Can you work these out from the model? Positions are in its coordinate system, mm. Face numbers are marked on the shaded views. A direction names the side the tool comes from. Give positions to 0.01 mm unless a question says otherwise; leave off trailing zeros. Loops run counter-clockwise (first coordinate to the right, second up) from the corner with the lowest first, then second, coordinate; pieces in that order, holes last. Notation, with made-up numbers: (-23, 85) -> (5, 85) arc R17 ccw to (5, 94) -> close; hole circle Ø11 at (47.5, 20.25). An arc over 180 degrees is marked (long way). Use CSV: the item, a comma, the result in double quotes.
from build123d import *

# Parameters (mm, degrees)
BOSS_EXTRUDE1_DEPTH       = 3
SKETCH2_W                 = 10
SKETCH2_H                 = 4.5
BOSS_EXTRUDE2_DEPTH       = 5
M2X0_4_TAPPED_HOLE1_D     = 1.6
M2X0_4_TAPPED_HOLE1_DEPTH = 5.2
M2X0_4_TAPPED_HOLE1_TIP   = 0.480688495
M3X0_5_TAPPED_HOLE1_D     = 2.5
M14_CLEARANCE_HOLE1_D     = 16
FILLET1_R                 = 1.749999932


with BuildPart() as part:
    # Sketch1 → Boss-Extrude1 (new body)
    with BuildSketch(Plane.XZ):
        with BuildLine():
            Line((-5, 5.422252789), (-5, 0))
            Line((-5, 0), (5, 0))
            Line((5, 0), (5, 5.422252789))
            ThreePointArc((5, 5.422252789), (0, 23), (-5, 5.422252789))
        make_face()
    extrude(amount=-BOSS_EXTRUDE1_DEPTH)

    # Sketch2 → Boss-Extrude2 (add)
    with BuildSketch(Plane.XZ):
        with Locations((0, 2.25)):
            Rectangle(SKETCH2_W, SKETCH2_H)
    extrude(amount=BOSS_EXTRUDE2_DEPTH)

    # M2x0.4 Tapped Hole1
    with Locations(Plane(origin=(0, 0, 0), x_dir=(-1, 0, 0), z_dir=(0, 0, -1))):
        with Locations((-3, 1)):
            Hole(M2X0_4_TAPPED_HOLE1_D / 2, depth=M2X0_4_TAPPED_HOLE1_DEPTH)
            with Locations((0, 0, -(M2X0_4_TAPPED_HOLE1_DEPTH + M2X0_4_TAPPED_HOLE1_TIP / 2))):  # 118° drill point
                Cone(0, M2X0_4_TAPPED_HOLE1_D / 2, M2X0_4_TAPPED_HOLE1_TIP, mode=Mode.SUBTRACT)

    # M3x0.5 Tapped Hole1 (through all)
    with Locations(Plane.XY.offset(4.5)):
        with Locations((-1.5, -2)):
            Hole(M3X0_5_TAPPED_HOLE1_D / 2)

    # M14 Clearance Hole1 (through all)
    with Locations(Plane(origin=(0, 0, 0), x_dir=(-1, 0, 0), z_dir=(0, -1, 0))):
        with Locations((0, -13.5)):
            Hole(M14_CLEARANCE_HOLE1_D / 2)

    # Fillet1
    fillet1_edges = [part.edges().sort_by_distance(p)[0] for p in [
        (-5, 1.5, 5.422252789),
        (5, 1.5, 5.422252789),
    ]]
    fillet(fillet1_edges, radius=FILLET1_R)


solid = part.part
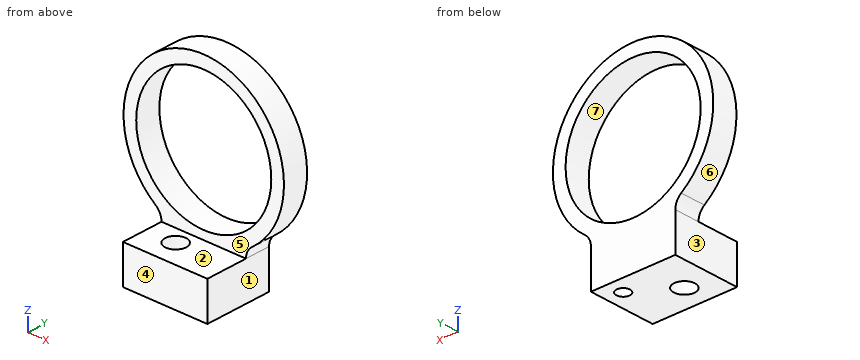
(1) If we section it at C-C, the plane z = 13.5: Write out the boundary of the cut face in (x, y), then the cut area to 3 significant figures.
Answer sheet:
outline,"(-9.5, 0) -> (-8, 0) -> (-8, 3) -> (-9.5, 3) -> close; (8, 0) -> (9.5, 0) -> (9.5, 3) -> (8, 3) -> close"
area,"9.00 mm2"
(2) Which directions (+Z, -Z, +X, -X, +Y, -Y) give clear straight access to the entire face, cutting with the end or side of a thin tool? Please do the marked faces 1, 2, 3 and 4.
Answer sheet:
face 1,"-Z, +X, +Y, -Y"
face 2,"+Z, +X, -X, -Y"
face 3,"-Z, -X, +Y, -Y"
face 4,"+Z, -Z, +X, -X, -Y"
(3) If we section it at A-A, the plane x = 0: Write out the boundary of the cut face in (y, z), then the cut area to 3 significant figures.
Answer sheet:
outline,"(-5, 0) -> (3, 0) -> (3, 5.5) -> (0, 5.5) -> (0, 4.5) -> (-5, 4.5) -> close; (0, 21.5) -> (3, 21.5) -> (3, 23) -> (0, 23) -> close"
area,"43.5 mm2"
(4) If we section it at D-D, the plane z = 1.5: Write out the boundary of the cut face in (x, y).
Answer sheet:
outline,"(-5, -5) -> (5, -5) -> (5, 3) -> (-5, 3) -> close; hole circle Ø2.5 at (-1.5, -2); hole circle Ø1.6 at (3, 1)"
(5) We'd pull the mould along Z, two halves only. Please class the marked faces 5, 6 and 7: released by +Z, released by -Z, zero draft, split by the parting line, or undercut.
Answer sheet:
face 5,"zero draft"
face 6,"split by the parting line"
face 7,"undercut"
(6) Will these pins go through, and if not, where does the flat tip stop? pin 1 Ø4 at (x, y) = (0, -1.5) entering from +Z; pin 2 Ø5.5 at (x, z) = (-3, 14) entering from -Y; pin 3 Ø2.5 at (y, z) = (-1, 3) entering from -X; pin 4 Ø1.3 at (x, y) = (3, 1) entering from +Z.
Answer sheet:
pin 1,"stops at z = 23"
pin 2,"passes through"
pin 3,"stops at x = -5"
pin 4,"stops at z = 22.7"
(7) If I drill on L1, parallel to Y at x = -1.5, z = 0.9; L2, parallel to X at y = 1, z = 2.15; L3, parallel to Y at x = 3, z = 1.45, over which ranges is the centre line in solid material (lowest first)? Write a range as from..to.
Answer sheet:
L1,"y = -5..-3.25, -0.75..3"
L2,"x = -5..2.2, 3.8..5"
L3,"y = -5..0.2, 1.8..3"
(8) If we section it at B-B, the plane y = -1: Write out the boundary of the cut face in (x, z), then the cut area to 4 significant figures.
Answer sheet:
outline,"(-5, 0) -> (-2.25, 0) -> (-2.25, 4.5) -> (-5, 4.5) -> close; (-0.75, 0) -> (5, 0) -> (5, 4.5) -> (-0.75, 4.5) -> close"
area,"38.25 mm2"
